Check sheet for the modelled part. Datum: model origin and axes. Units: mm. Face numbers are marked on the shaded views. A direction names the side the tool comes from. Round coordinates to 2 decimals unless told otherwise and drop trailing zeros. Order: outer loops, then holes, each group sorted by start corner. A loop starts at its lowest first (then second) coordinate and runs counter-clockwise, first axis right, second up. Notation, with made-up numbers: (11.25, -21) -> (58.25, -21) arc R23 cw to (58.25, -5) -> close; hole circle Ø9 at (24, 66). An arc over 180 degrees is marked (long way). Answer in a Markdown table with one row per item. Add a question column.
1. Sectioned sample at A-A, the plane y = -501. Record the boundary of the cut face in (x, z), then the cut area to 3 significant figures.
2. Depth check by flat-ended pin: P1, Ø12, axis at x = 2137, z = 2297, coming from the +Y side; P2, Ø10, axis at y = -498.5, z = 2291.5, coming from the +X side; P3, Ø2, axis at x = 2134.5, z = 2313, coming from the -Y side; P4, Ø1, axis at x = 2141.5, z = 2318, coming from the +Y side. Enter the tip coordinate at first touch or a pass-through.
3. Material ranges on L1, parallel to Z at x = 2148, y = -490; L2, parallel to X at y = -547.5, z = 2287; L3, parallel to Y at x = 2143.5, z = 2289, recorded low to high. Write a range as from..to.
4. Access from +Z, -Z, +X, -X, +Y, -Y to the whole of each face (thin tool, end or side, straight path). Record for the marked faces 1, 2, 3, 4 and 5.
5. Sectioned sample at C-C, the plane z = 2300.5. Record the boundary of the cut face in (x, y).
6. Sectioned sample at B-B, the plane x = 2127. Record the boundary of the cut face in (y, z).
7. Sectioned sample at D-D, the plane x = 2157. Record the boundary of the cut face in (y, z), then the cut area to 3 significant figures.
8. Draft check along Z on the marked faces 6, 7 and 8. Enter one of: +Z half, -Z half, draft (parallel to the pull), parting line (faces both ways), or undercut.
```python
from build123d import *

# Parameters (mm, degrees)
PAD005_DEPTH    = 45
POCKET002_DEPTH = 10.001
PAD006_DEPTH    = 10


with BuildPart() as part:
    # Sketch012 → Pad005 (new body, symmetric)
    with BuildSketch(Plane(origin=(0, -526, 0), x_dir=(1, 0, 0), z_dir=(0, 1, 0))):
        Polygon((2110, -2335), (2110, -2260), (2160, -2260), (2160, -2270), (2120, -2270), (2120, -2335), align=None)
    extrude(amount=PAD005_DEPTH, both=True)

    # Sketch013 (on Face5 of Pad005) → Pocket002 (cut, through all)
    with BuildSketch(Plane(origin=(2120, -526, 0), x_dir=(0, 0, -1), z_dir=(1, 0, 0))):
        with BuildLine():
            ThreePointArc((-2310, -20), (-2315, -25), (-2310, -30))
            Line((-2310, -30), (-2295, -30))
            ThreePointArc((-2295, -30), (-2290, -25), (-2295, -20))
            Line((-2310, -20), (-2295, -20))
        make_face()
        with BuildLine():
            ThreePointArc((-2310, 30), (-2315, 25), (-2310, 20))
            Line((-2310, 20), (-2295, 20))
            ThreePointArc((-2295, 20), (-2290, 25), (-2295, 30))
            Line((-2310, 30), (-2295, 30))
        make_face()
    extrude(amount=-POCKET002_DEPTH, mode=Mode.SUBTRACT)

    # Sketch003 (on DatumPlane) → Pad006 (join, symmetric)
    with BuildSketch(Plane(origin=(0, -526, 0), x_dir=(-1, 0, 0), z_dir=(0, 1, 0))):
        Polygon((-2160, 2270), (-2160, 2280), (-2130, 2335), (-2120, 2335), (-2120, 2270), align=None)
    extrude(amount=PAD006_DEPTH, both=True)


solid = part.part
```
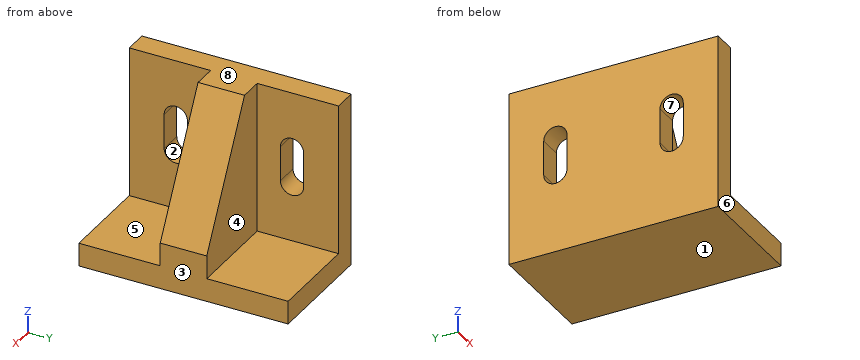
Answer key:
| question | item | result |
|---|---|---|
| 1 | outline | (2110, 2260) -> (2160, 2260) -> (2160, 2270) -> (2120, 2270) -> (2120, 2290) -> (2110, 2290) -> close; (2110, 2315) -> (2120, 2315) -> (2120, 2335) -> (2110, 2335) -> close |
| 1 | area | 900 mm² |
| 2 | P1 | stops at y = -516 |
| 2 | P2 | stops at x = 2120 |
| 2 | P3 | stops at y = -536 |
| 2 | P4 | passes through |
| 3 | L1 | z = 2260..2270 |
| 3 | L2 | x = 2110..2120 |
| 3 | L3 | y = -536..-516 |
| 4 | face 1 | -Z, +X, -X, +Y, -Y |
| 4 | face 2 | +X, -X |
| 4 | face 3 | +Z, -Z, +X, +Y, -Y |
| 4 | face 4 | +Z, +X, +Y |
| 4 | face 5 | +Z, +X, -Y |
| 5 | outline | (2110, -571) -> (2120, -571) -> (2120, -556) -> (2110, -556) -> close; (2110, -546) -> (2120, -546) -> (2120, -536) -> (2148.82, -536) -> (2148.82, -516) -> (2120, -516) -> (2120, -506) -> (2110, -506) -> close; (2110, -496) -> (2120, -496) -> (2120, -481) -> (2110, -481) -> close |
| 6 | outline | (-571, 2260) -> (-481, 2260) -> (-481, 2270) -> (-516, 2270) -> (-516, 2335) -> (-536, 2335) -> (-536, 2270) -> (-571, 2270) -> close |
| 7 | outline | (-571, 2260) -> (-481, 2260) -> (-481, 2270) -> (-516, 2270) -> (-516, 2285.5) -> (-536, 2285.5) -> (-536, 2270) -> (-571, 2270) -> close |
| 7 | area | 1,210 mm² |
| 8 | face 6 | draft |
| 8 | face 7 | undercut |
| 8 | face 8 | +Z half |
